Geometry: final body of the model. Coordinates: model frame, mm. Face numbers are marked on the shaded views. A direction names the side the tool comes from. Coordinates: 2 decimals unless noted, no trailing zeros. Write each loop counter-clockwise with the first axis right and the second up, starting at its lowest first coordinate (ties: lowest second). Pieces come first, ordered by that corner, then holes. Notation, with made-up numbers: (81.5, -21.5) -> (114.5, -21.5) arc R32 ccw to (114.5, 13.5) -> close; hole circle Ø8 at (72, 6). An arc over 180 degrees is marked (long way). One line per item, written item: value.
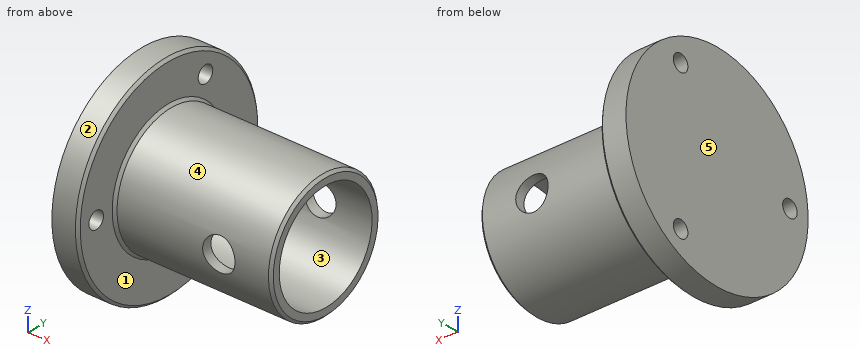
```python
from build123d import *

# Parameters (mm, degrees)
SKETCH_1_R               = 20
EXTRUDE_1_DEPTH          = 5
SKETCH_6_R               = 12
EXTRUDE_2_DEPTH          = 30
SKETCH_7_R               = 10.2
CUT_EXTRUDE_2_DEPTH      = 30
CHAMFER_1_SIZE           = 0.5
CUT_EXTRUDE_3_DEPTH      = 46
CUT_EXTRUDE_3_DEPTH_BACK = 46
SKETCH_8_R               = 3.1
CHAMFER_2_SIZE           = 0.5
CHAMFER_3_SIZE           = 0.5
SKETCH_9_R               = 1.6
CUT_EXTRUDE_4_DEPTH      = 10


with BuildPart() as part:
    # 草图1 → 凸台-拉伸1 (new body)
    with BuildSketch(Plane(origin=(0, 0, 0), x_dir=(0, 0, -1), z_dir=(1, 0, 0))):
        Circle(SKETCH_1_R)
    extrude(amount=EXTRUDE_1_DEPTH)

    # 草图6 → 凸台-拉伸2 (add)
    with BuildSketch(Plane(origin=(5, 0, 0), x_dir=(0, 0, -1), z_dir=(1, 0, 0))):
        Circle(SKETCH_6_R)
    extrude(amount=EXTRUDE_2_DEPTH)

    # 草图7 → 切除-拉伸2 (cut)
    with BuildSketch(Plane(origin=(35, 0, 0), x_dir=(0, 0, -1), z_dir=(1, 0, 0))):
        Circle(SKETCH_7_R)
    extrude(amount=-CUT_EXTRUDE_2_DEPTH, mode=Mode.SUBTRACT)

    # 倒角1
    chamfer_1_edges = [part.edges().sort_by_distance(p)[0] for p in [
        (35, 0, 12),
    ]]
    chamfer(chamfer_1_edges, length=CHAMFER_1_SIZE)

    # 草图8 → 切除-拉伸3 (cut, two sides: drawn at the far end of the back side and taken through both)
    with BuildSketch(Plane(origin=(0, 0, 0), x_dir=(1, 0, 0), z_dir=(0, 1, 0)).offset(-CUT_EXTRUDE_3_DEPTH_BACK)):
        with Locations(Location((25, 0, 0), (0, 0, 90))):
            Circle(SKETCH_8_R)
    extrude(amount=CUT_EXTRUDE_3_DEPTH + CUT_EXTRUDE_3_DEPTH_BACK, mode=Mode.SUBTRACT)

    # 倒角2
    chamfer_2_edges = [part.edges().sort_by_distance(p)[0] for p in [
        (5, 0, 20),
    ]]
    chamfer(chamfer_2_edges, length=CHAMFER_2_SIZE)

    # 倒角3
    chamfer_3_edges = [part.edges().sort_by_distance(p)[0] for p in [
        (5, 0, 12),
    ]]
    chamfer(chamfer_3_edges, length=CHAMFER_3_SIZE)

    # 草图9 → 切除-拉伸4 (cut)
    with BuildSketch(Plane.ZY):
        with Locations((-13.856406461, 8)):
            Circle(SKETCH_9_R)
        with Locations((13.856406461, 8)):
            Circle(SKETCH_9_R)
        with Locations((0, -16)):
            Circle(SKETCH_9_R)
    extrude(amount=-CUT_EXTRUDE_4_DEPTH, mode=Mode.SUBTRACT)


solid = part.part
```
(1) Line query: line 1 (Z direction, x = 20, y = -0.5); line 2 (X direction, y = 8.5, z = -2.5). Output: solid intervals per line, ascending. Write a range as [from, to].
Responses:
line 1: z = [-11.99, -10.19], [10.19, 11.99]
line 2: x = [0, 5]
(2) Section B-B (x = 29). Return the cut outline in (y, z).
Responses:
outline: circle Ø24 at (0, 0); hole circle Ø20.4 at (0, 0)
(3) Reachability of the marked faces 1 and 2 from +Z, -Z, +X, -X, +Y, -Y: full face, straight path, thin tool, end or side. Return the list, or none.
Responses:
face 1: +X
face 2: +X, -X
(4) Pull-direction query (Y, two-part tool) for the marked faces 3, 4 and 5; classes: released by +Y, released by -Y, zero draft, split by the parting line, or undercut.
Responses:
face 3: undercut
face 4: split by the parting line
face 5: zero draft
(5) First-contact query: pin 1 (3 mm diameter, centred on x = 11, y = -14.5, fed in from -Z); pin 2 (4 mm diameter, centred on y = 10, z = 1, fed in from -X); pin 3 (4 mm diameter, centred on x = 31, z = -10, fed in from -Y); pin 4 (6 mm diameter, centred on y = 1, z = -3.5, fed in from +X). Flat tips, straight axial feed; report the tip coordinate or a pass-through.
Responses:
pin 1: passes through
pin 2: stops at x = 0
pin 3: stops at y = -8.94
pin 4: stops at x = 5
(6) Section A-A (z = 0). State how many separate pieces and enclosed holes the cut face has, then the cut area to 3 significant figures.
Responses:
separate pieces: 4
enclosed holes: 0
area: 269 mm2
